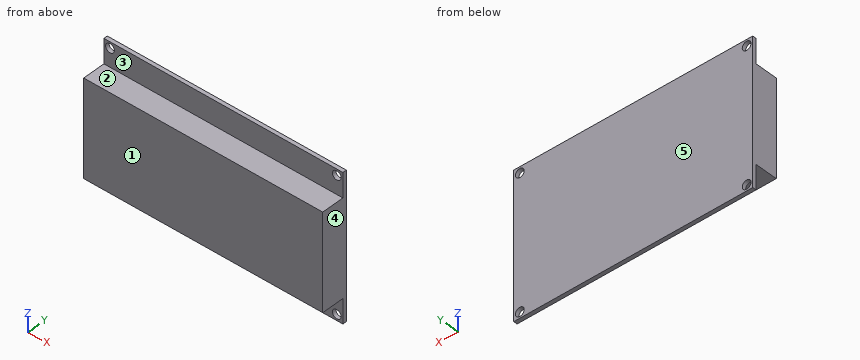
```python
from build123d import *

# Parameters (mm, degrees)
F0_W     = 98
F0_H     = 59.5
F1_DEPTH = 1.55
F2_W     = 98
F2_H     = 39.5
F3_DEPTH = 9.25
F4_R     = 1.8
F5_DEPTH = 25


with BuildPart() as f1:
    # F0 (on Front) → F1 (new body)
    with BuildSketch(Plane.XZ):
        Rectangle(F0_W, F0_H)
    extrude(amount=F1_DEPTH)

    # F2 (on face) → F3 (join)
    with BuildSketch(Plane.XZ.offset(1.55)):
        Rectangle(F2_W, F2_H)
    extrude(amount=F3_DEPTH)

    # F4 (on face) → F5 (cut)
    with BuildSketch(Plane.XZ.offset(1.55)):
        with Locations((-46.5, 27.25)):
            Circle(F4_R)
        with Locations((-46.5, -27.25)):
            Circle(F4_R)
        with Locations((46.5, -27.25)):
            Circle(F4_R)
        with Locations((46.5, 27.25)):
            Circle(F4_R)
    extrude(amount=-F5_DEPTH, mode=Mode.SUBTRACT)


solid = f1.part
```
Design review of the part built by this model. Coordinates are the model's own, in mm. Face numbers are marked on the shaded views. A direction names the side the tool comes from. Give positions to 0.01 mm unless a question says otherwise; leave off trailing zeros. Order: outer loops, then holes, each group sorted by start corner. A loop starts at its lowest first (then second) coordinate and runs counter-clockwise, first axis right, second up. Notation, with made-up numbers: (-38.5, 55.5) -> (1.5, 55.5) arc R15 ccw to (1.5, 67.5) -> close; hole circle Ø1 at (43, 53). An arc over 180 degrees is marked (long way). Write item = value, one per line. Start each with the question number.
(1) Mouldability with a two-part tool opening along Y and no side actions: class the marked faces 3, 4 and 5 as +Y half, -Y half, draft (parallel to the pull), parting line (faces both ways), or undercut.
(2) To check wall thickness, follow line 1 along Z through (x, y) = (46.5, -0.85); line 2 along Z through (x, y) = (-6, -2.5); line 3 along Y through (x, z) = (-3, 26.5). State the ranges of each line that lie inside material, in increasing order.
(3) For the marked faces 1 and 2, list the 3-axis set-ups (+Z, -Z, +X, -X, +Y, -Y) from which the entire face can be reached by the end or side of a thin tool; tool diameter is ignored.
(4) For pin 1 (5 mm diameter, centred on x = 20.5, z = 26.5, fed in from -Y); pin 2 (4.5 mm diameter, centred on x = 21.5, y = -4.5, fed in from +Z); pin 3 (2 mm diameter, centred on x = 46.5, z = -27.25, fed in from -Y), all flat-tipped, find the tip position at first contact; note any pin that passes through.
(5) We need section D-D on y = -9.25. Write out the cut boundary in (x, z), plus the area to 3 significant figures.
(6) We need section B-B on x = -46.5. Write out the cut boundary in (y, z).
(7) We need section A-A on z = -27.25. Write out the cut boundary in (x, y).
(8) We need section C-C on x = -11. Write out the cut boundary in (y, z).
Numbers:
q1.face_3 = -Y half
q1.face_4 = draft
q1.face_5 = +Y half
q2.line_1 = -29.75 to -29.05, -25.45 to 25.45, 29.05 to 29.75
q2.line_2 = -19.75 to 19.75
q2.line_3 = -1.55 to 0
q3.face_1 = +Z, -Z, +X, -X, -Y
q3.face_2 = +Z, +X, -X, -Y
q4.pin_1 = -1.55
q4.pin_2 = 19.75
q4.pin_3 = through
q5.outline = (-49, -19.75) -> (49, -19.75) -> (49, 19.75) -> (-49, 19.75) -> close
q5.area = 3,870 mm^2
q6.outline = (-10.8, -19.75) -> (-1.55, -19.75) -> (-1.55, -25.45) -> (0, -25.45) -> (0, 25.45) -> (-1.55, 25.45) -> (-1.55, 19.75) -> (-10.8, 19.75) -> close; (-1.55, -29.75) -> (0, -29.75) -> (0, -29.05) -> (-1.55, -29.05) -> close; (-1.55, 29.05) -> (0, 29.05) -> (0, 29.75) -> (-1.55, 29.75) -> close
q7.outline = (-49, -1.55) -> (-48.3, -1.55) -> (-48.3, 0) -> (-49, 0) -> close; (-44.7, -1.55) -> (44.7, -1.55) -> (44.7, 0) -> (-44.7, 0) -> close; (48.3, -1.55) -> (49, -1.55) -> (49, 0) -> (48.3, 0) -> close
q8.outline = (-10.8, -19.75) -> (-1.55, -19.75) -> (-1.55, -29.75) -> (0, -29.75) -> (0, 29.75) -> (-1.55, 29.75) -> (-1.55, 19.75) -> (-10.8, 19.75) -> close
